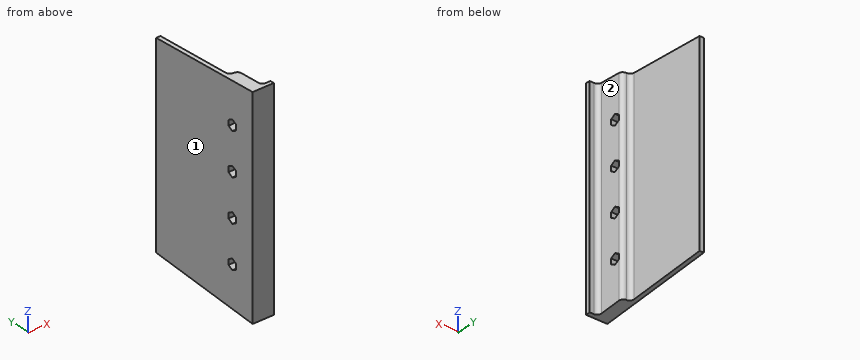
```python
from build123d import *

# Parameters (mm, degrees)
GENERAL_EXTRUDE_DEPTH             = 125.3
ROUNDING_R                        = 5
ROLLER_HOLDERS_DEPTH              = 130.325519523
SKETCH5_W                         = 5
SKETCH5_H                         = 250.6
GUARD_RAIL_DEPTH                  = 100
GUARD_RAIL_SUPPORT_FILLET_R       = 5
SLANT_FOR_INPUT_FROM_SORTER_DEPTH = 175.642749635


with BuildPart() as part:
    # Sketch2 → General extrude (new, symmetric)
    with BuildSketch(Plane.XY):
        Polygon((-12.5, 20), (-12.5, -20), (12.5, -20), (12.5, -15), (2.5, -15), (2.5, 20), align=None)
    extrude(amount=GENERAL_EXTRUDE_DEPTH, both=True)

    # Rounding
    rounding_edges = [part.edges().sort_by_distance(p)[0] for p in [
        (2.5, 20, 0),
        (2.5, -15, 0),
    ]]
    fillet(rounding_edges, radius=ROUNDING_R)

    # Sketch3 → Roller holders (cut, through all)
    with BuildSketch(Plane.ZY.offset(12.5)):
        Polygon((-72.004573519, 4), (-68.829147039, 9.5), (-72.004573519, 15), (-78.355426481, 15), (-81.530852961, 9.5), (-78.355426481, 4), align=None)
        Polygon((-21.884573519, 4), (-18.709147039, 9.5), (-21.884573519, 15), (-28.235426481, 15), (-31.410852961, 9.5), (-28.235426481, 4), align=None)
        Polygon((28.235426481, 4), (31.410852961, 9.5), (28.235426481, 15), (21.884573519, 15), (18.709147039, 9.5), (21.884573519, 4), align=None)
        Polygon((78.355426481, 4), (81.530852961, 9.5), (78.355426481, 15), (72.004573519, 15), (68.829147039, 9.5), (72.004573519, 4), align=None)
    extrude(amount=-ROLLER_HOLDERS_DEPTH, mode=Mode.SUBTRACT)

    # Sketch5 → Guard rail (add)
    with BuildSketch(Plane(origin=(0, 20, 0), x_dir=(1, 0, 0), z_dir=(0, 1, 0))):
        with Locations((-10, 0)):
            Rectangle(SKETCH5_W, SKETCH5_H)
    extrude(amount=GUARD_RAIL_DEPTH)

    # Guard rail support fillet
    guard_rail_support_fillet_edges = [part.edges().sort_by_distance(p)[0] for p in [
        (-7.5, 20, 0),
    ]]
    fillet(guard_rail_support_fillet_edges, radius=GUARD_RAIL_SUPPORT_FILLET_R - 0.0001)  # a hair under: the kernel refuses the full size

    # Sketch6 → Slant for input from sorter (cut, symmetric)
    with BuildSketch(Plane(origin=(-7.5, 0, 0), x_dir=(0, 0, -1), z_dir=(1, 0, 0))):
        Polygon((-125.3, 120), (-125.3, -20), (-116.093807983, 120), align=None)
    slant_for_input_from_sorter = extrude(amount=SLANT_FOR_INPUT_FROM_SORTER_DEPTH, both=True, mode=Mode.SUBTRACT)

    # Mirror of cut above (since same part is used on both sides): Slant for input from sorter across plane
    add(slant_for_input_from_sorter.mirror(Plane.XY), mode=Mode.SUBTRACT)


solid = part.part
```
CAD build for the part. Positions are in the model's coordinates, mm. Face numbers are marked on the shaded views. A direction names the side the tool comes from. Round coordinates to 2 decimals unless told otherwise and drop trailing zeros. Order: outer loops, then holes, each group sorted by start corner. A loop starts at its lowest first (then second) coordinate and runs counter-clockwise, first axis right, second up. Notation, with made-up numbers: (9, 10) - (45, 10) arc R25 ccw to (45, 27) - close; hole circle Ø4 at (7, -37.5). An arc over 180 degrees is marked (long way). Answer in a Markdown table with one row per item. Add a question column.
(1) Probe L1, parallel to Z at x = -9, y = 8; L2, parallel to X at y = 74, z = -52.5; L3, parallel to Z at x = -7.25, y = 6. List the from-to ranges inside material, lowest first. Write a range as [from, to].
(2) Band-saw the part on B-B on y = 110.5. List the corners of the cut face in (x, z).
(3) Band-saw the part on C-C on y = 49. List the corners of the cut face in (x, z).
(4) Drop flat-ended pins along their axis: pin 1 Ø10 at (x, y) = (6, 18) entering from -Z; pin 2 Ø3 at (x, z) = (7.5, 72.5) entering from +Y; pin 3 Ø1.5 at (y, z) = (14.5, 89) entering from +X. Give the stop position or say it passes through.
(5) 3-axis set-ups, long thin cutter, end or side, ignore diameter. For the marked faces 1 and 2: which of +Z, -Z, +X, -X, +Y, -Y reach the whole face in a straight line?
Data:
| question | item | result |
|---|---|---|
| 1 | L1 | z = [-123.46, -80.66], [-69.7, -30.54], [-19.58, 19.58], [30.54, 69.7], [80.66, 123.46] |
| 1 | L2 | x = [-12.5, -7.5] |
| 1 | L3 | z = [-123.59, -79.51], [-70.85, -29.39], [-20.73, 20.73], [29.39, 70.85], [79.51, 123.59] |
| 2 | outline | (-12.5, -116.72) - (-7.5, -116.72) - (-7.5, 116.72) - (-12.5, 116.72) - close |
| 3 | outline | (-12.5, -120.76) - (-7.5, -120.76) - (-7.5, 120.76) - (-12.5, 120.76) - close |
| 4 | pin 1 | stops at z = -123.04 |
| 4 | pin 2 | stops at y = -14.77 |
| 4 | pin 3 | stops at x = 2.5 |
| 5 | face 1 | +Z, -Z, -X, +Y, -Y |
| 5 | face 2 | +Z, -Z, +X, +Y |
